The figure shows three views and two pictorial views of one solid part (mm, origin at its lowest corner). Answer the questions. A direction names the side the tool comes from. Coordinates: 2 decimals unless noted, no trailing zeros. Order: outer loops, then holes, each group sorted by start corner. A loop starts at its lowest first (then second) coordinate and runs counter-clockwise, first axis right, second up. Notation, with made-up numbers: M 83,88 L 131,88 A20 ccw 131,106 Z; hole C 40.5,41.5 d6. An arc over 180 degrees is marked long. Use a Markdown table: item, result.
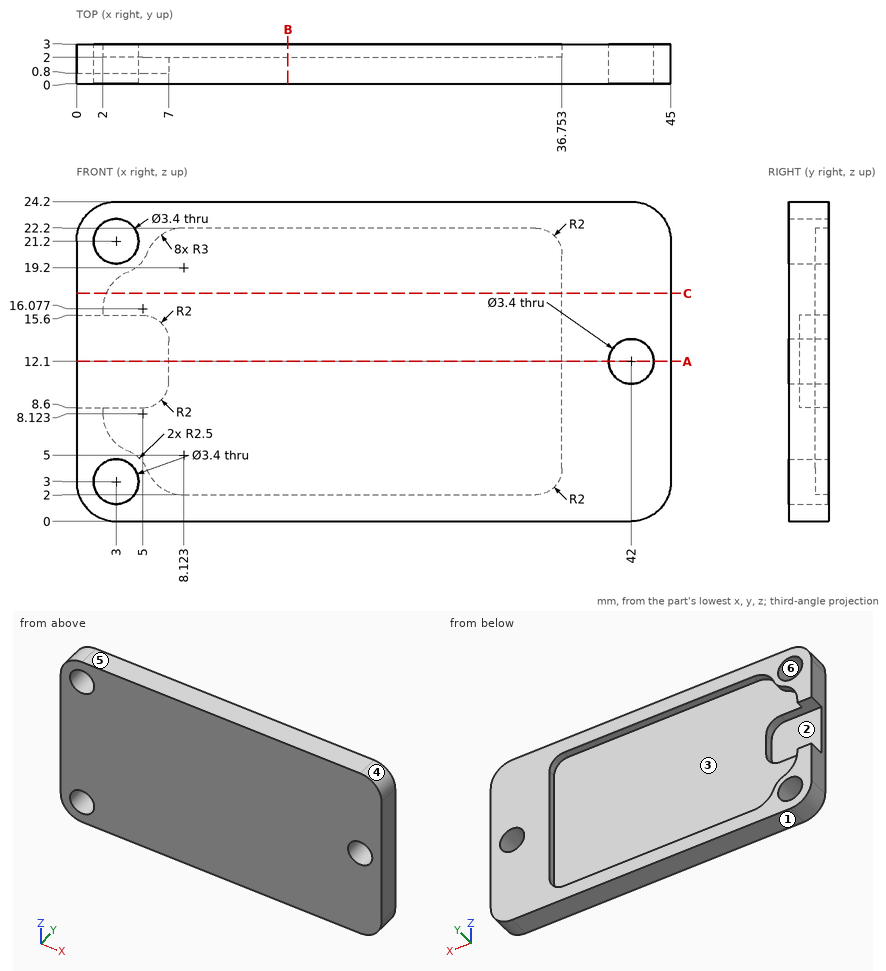
1. Section A-A on z = 12.1 is taken. Determine the outline of the cut face in (x, y).
Answers below:
| item | result |
|---|---|
| outline | M 0,0 L 40.3,0 L 40.3,3 L 36.75,3 L 36.75,2 L 7,2 L 7,0.8 L 0,0.8 Z; M 43.7,0 L 45,0 L 45,3 L 43.7,3 Z |
2. For the marked faces 1, 2 and 3, determine the directions among +Z, -Z, +X, -X, +Y, -Y from which every point of the face is accessible in a straight line to the end or side of a thin tool.
Answers below:
| item | result |
|---|---|
| face 1 | -Z, +X, -X, +Y, -Y |
| face 2 | -X, +Y |
| face 3 | +Y |
3. For a pull along X with two mould halves and no side action, classify the marked faces 4, 5 and 6 as +X half, -X half, draft (parallel to the pull), parting line (faces both ways), or undercut.
Answers below:
| item | result |
|---|---|
| face 4 | +X half |
| face 5 | draft |
| face 6 | undercut |
4. Find the intervals of material crossed by probe 1 along X at (y, z) = (1.4, 12.1); probe 2 along Z at (x, y) = (42, 1.75); probe 3 along Z at (x, y) = (21, 2.75), in increasing order.
Answers below:
| item | result |
|---|---|
| probe 1 | 7 to 40.3, 43.7 to 45 |
| probe 2 | 0 to 10.4, 13.8 to 24.2 |
| probe 3 | 0 to 2, 22.2 to 24.2 |
5. Flat-ended cylindrical pins translate along their axes: P1, Ø0.5, axis at y = 2.5, z = 9, coming from the -X side; P2, Ø1, axis at y = 1.5, z = 11.5, coming from the -X side. Find the tip coordinate at first contact, or state that the pin passes through.
Answers below:
| item | result |
|---|---|
| P1 | x = 36.75 |
| P2 | x = 7 |
6. Section C-C on z = 17.25 is taken. Determine the outline of the cut face in (x, y).
Answers below:
| item | result |
|---|---|
| outline | M 0,0 L 45,0 L 45,3 L 36.75,3 L 36.75,2 L 2.24,2 L 2.24,3 L 0,3 Z |
7. Section B-B on x = 16 is taken. Determine the outline of the cut face in (y, z).
Answers below:
| item | result |
|---|---|
| outline | M 0,0 L 3,0 L 3,2 L 2,2 L 2,22.2 L 3,22.2 L 3,24.2 L 0,24.2 Z |
